from build123d import *
from build123d.topology import SkipClean

# Parameters (mm, degrees)
SKETCH1_R           = 12.35
SKETCH1_R_2         = 10.35
BOSS_EXTRUDE1_DEPTH = 50
SKETCH2_R           = 9.85
BOSS_EXTRUDE2_DEPTH = 42
SKETCH2_3_R         = 9.85
BOSS_EXTRUDE3_DEPTH = 6
SKETCH1_2_R         = 10.35
CUT_EXTRUDE1_DEPTH  = 51


with BuildPart() as part:
    # Sketch1 → Boss-Extrude1 (new body)
    with BuildSketch(Plane.XY):
        Circle(SKETCH1_R)
        Circle(SKETCH1_R_2, mode=Mode.SUBTRACT)
    extrude(amount=BOSS_EXTRUDE1_DEPTH)



with BuildPart() as body_2:
    # Sketch2 → Boss-Extrude2 (new body)
    with BuildSketch(Plane(origin=(0, 11, 0), x_dir=(1, 0, 0), z_dir=(0, 1, 0))):
        with Locations(Location((0, -25, 0), (0, 0, 90))):
            Circle(SKETCH2_R)
    extrude(amount=BOSS_EXTRUDE2_DEPTH)


with BuildPart() as part_1:
    with SkipClean():  # the faces are left unmerged after this step: merging them gives an invalid solid
        add(part.part)

        add(body_2.part)  # Boss-Extrude3 merges body 2
        # Sketch2_3 → Boss-Extrude3 (add)
        with BuildSketch(Plane(origin=(0, 11, 0), x_dir=(1, 0, 0), z_dir=(0, 1, 0))):
            with Locations(Location((0, -25, 0), (0, 0, 270))):
                Circle(SKETCH2_3_R)
        extrude(amount=-BOSS_EXTRUDE3_DEPTH)

    # Sketch1_2 → Cut-Extrude1 (cut)
    with SkipClean():  # the faces are left unmerged after this step: merging them gives an invalid solid
        with BuildSketch(Plane.XY):
            Circle(SKETCH1_2_R)
        extrude(amount=CUT_EXTRUDE1_DEPTH, mode=Mode.SUBTRACT)


solid = part_1.part
CAD build for the part. Positions are in the model's coordinates, mm. A direction names the side the tool comes from. Give positions to 0.01 mm unless a question says otherwise; leave off trailing zeros. Write each loop counter-clockwise with the first axis right and the second up, starting at its lowest first coordinate (ties: lowest second). Pieces come first, ordered by that corner, then holes. Notation, with made-up numbers: (-9.5, -20.5) -> (45.5, -20.5) arc R18 ccw to (45.5, 0.5) -> close; hole circle Ø2 at (39, 38). An arc over 180 degrees is marked (long way). Return JSON: item names as keys, results as strings.
Item 1: Tool access for faces 1 (the flat face through (0, 53, 25)), 2 (the cylindrical face through (-2.677, -12.056, 24.65)): list every direction of +Z, -Z, +X, -X, +Y, -Y with a clear straight run to the whole face (end or side of a thin tool).
Answer below:
{"face 1": "+Z, -Z, +X, -X, +Y", "face 2": "none"}
Item 2: Band-saw the part on D-D (x = 4). List the corners of the cut face in (y, z).
Answer below:
{"outline": "(-11.68, 0) -> (-9.55, 0) -> (-9.55, 50) -> (-11.68, 50) -> close; (9.55, 0) -> (11.68, 0) -> (11.68, 16) -> (53, 16) -> (53, 34) -> (11.68, 34) -> (11.68, 50) -> (9.55, 50) -> close"}
Item 3: Drill centre lines: probe 1 along Y at (x, z) = (-0.5, 32.5); probe 2 along Y at (x, z) = (0, 13.5); probe 3 along X at (y, z) = (4, 21). Where is each one in solid material? Low to high.
Answer below:
{"probe 1": "y = -12.34 to -10.34, 10.34 to 53", "probe 2": "y = -12.35 to -10.35, 10.35 to 12.35", "probe 3": "x = -11.68 to -9.55, 9.55 to 11.68"}
Item 4: Band-saw the part on A-A (y = 0). List the corners of the cut face in (x, z), then the cut area to 3 significant figures.
Answer below:
{"outline": "(-12.35, 0) -> (-10.35, 0) -> (-10.35, 50) -> (-12.35, 50) -> close; (10.35, 0) -> (12.35, 0) -> (12.35, 50) -> (10.35, 50) -> close", "area": "200 mm2"}
Item 5: Drop flat-ended pins along their axis: pin 1 (4 mm diameter, centred on x = -2.5, y = 40.5, fed in from +Z); pin 2 (4 mm diameter, centred on x = 6.5, z = 11, fed in from +Y); pin 3 (4 mm diameter, centred on x = 8.5, y = 25.5, fed in from -Z). Give the stop position or say it passes through.
Answer below:
{"pin 1": "stops at z = 34.84", "pin 2": "stops at y = 11.5", "pin 3": "stops at z = 17.6"}
Item 6: Band-saw the part on B-B (x = 0). List the corners of the cut face in (y, z), then the cut area to 3 significant figures.
Answer below:
{"outline": "(-12.35, 0) -> (-10.35, 0) -> (-10.35, 50) -> (-12.35, 50) -> close; (10.35, 0) -> (12.35, 0) -> (12.35, 15.15) -> (53, 15.15) -> (53, 34.85) -> (12.35, 34.85) -> (12.35, 50) -> (10.35, 50) -> close", "area": "1,000 mm2"}
Item 7: Band-saw the part on C-C (z = 25). List the corners of the cut face in (x, y), then the cut area to 3 significant figures.
Answer below:
{"outline": "(-9.85, 7.45) arc R12.35 ccw (long way) to (9.85, 7.45) -> (9.85, 53) -> (-9.85, 53) -> close; hole circle Ø20.7 at (0, 0)", "area": "973 mm2"}
